Can you work these out from the model? Positions are in its coordinate system, mm. A direction names the side the tool comes from. Round coordinates to 2 decimals unless told otherwise and drop trailing zeros. Loops run counter-clockwise (first coordinate to the right, second up) from the corner with the lowest first, then second, coordinate; pieces in that order, holes last.
```python
from build123d import *

# Parameters (mm, degrees)
SKETCH1_R           = 2.5
BOSS_EXTRUDE1_DEPTH = 7.5


with BuildPart() as part:
    # Sketch1 → Boss-Extrude1 (new body)
    # profile 1 of 2: a face of its own
    with BuildSketch(Plane.XY):
        with BuildLine():
            ThreePointArc((47, 4), (55, 0), (47, -4))
            Line((47, -4), (-47, -4))
            ThreePointArc((-47, -4), (-55, 0), (-47, 4))
            Line((-47, 4), (47, 4))
        make_face()
        Circle(SKETCH1_R, mode=Mode.SUBTRACT)
        with BuildLine():
            ThreePointArc((52.5, 1.5), (52.207106781, 2.207106781), (51.5, 2.5))
            Line((51.5, 2.5), (48.5, 2.5))
            ThreePointArc((48.5, 2.5), (47.792893219, 2.207106781), (47.5, 1.5))
            Line((47.5, 1.5), (47.5, -1.5))
            ThreePointArc((47.5, -1.5), (47.792893219, -2.207106781), (48.5, -2.5))
            Line((48.5, -2.5), (51.5, -2.5))
            ThreePointArc((51.5, -2.5), (52.207106781, -2.207106781), (52.5, -1.5))
            Line((52.5, -1.5), (52.5, 1.5))
        make_face(mode=Mode.SUBTRACT)
        with BuildLine():
            Line((-52.5, -1.5), (-52.5, 1.5))
            ThreePointArc((-52.5, 1.5), (-52.207106781, 2.207106781), (-51.5, 2.5))
            Line((-51.5, 2.5), (-48.5, 2.5))
            ThreePointArc((-48.5, 2.5), (-47.792893219, 2.207106781), (-47.5, 1.5))
            Line((-47.5, 1.5), (-47.5, -1.5))
            ThreePointArc((-47.5, -1.5), (-47.792893219, -2.207106781), (-48.5, -2.5))
            Line((-48.5, -2.5), (-51.5, -2.5))
            ThreePointArc((-51.5, -2.5), (-52.207106781, -2.207106781), (-52.5, -1.5))
        make_face(mode=Mode.SUBTRACT)
    # profile 2 of 2: a face of its own
    with BuildSketch(Plane.XY):
        Circle(SKETCH1_R)
    extrude(amount=BOSS_EXTRUDE1_DEPTH)


solid = part.part
```
(1) Which directions (+Z, -Z, +X, -X, +Y, -Y) give clear straight access to the entire face, cutting with the end or side of a thin tool? Please do faces 1 (the flat face through (-1, 4, 4)), 2 (the flat face through (-50, -2.5, 4)), 3 (the flat face through (1, -4, 4)).
(2) Suppose I cut it at A-A (x = 50). Write out the boundary of the cut face in (y, z).
(3) If I drill on line 1 (Y direction, x = 3.5, z = 1); line 2 (X direction, y = -0.5, z = 5.25); line 3 (Y direction, x = 49, z = 4), over which ranges is the centre line in solid material (lowest first)?
(4) Suppose I cut it at D-D (x = -6). Write out the boundary of the cut face in (y, z).
(5) We'd pull the mould along X, two halves only. Please class faces 4 (the flat face through (1, 0, 7.5)), 5 (the flat face through (47.5, 0, 4)), 6 (the flat face through (52.5, 0, 4)): released by +X, released by -X, zero draft, split by the parting line, or undercut.
(6) Suppose I cut it at C-C (z = 5.5). Write out the boundary of the cut face in (x, y).
(7) Suppose I cut it at B-B (y = 0). Write out the boundary of the cut face in (x, z), then the cut area to 3 significant figures.
(8) For pin 1 (1 mm diameter, centred on x = 24.5, y = 3, fed in from -Z); pin 2 (2 mm diameter, centred on x = -20, z = 4, fed in from +Y), each with a flat end and sliding along its axis, tell me the tip position at first contact or that it passes through.
Check result:
1. face 1: +Z, -Z, +Y
1. face 2: +Z, -Z
1. face 3: +Z, -Z, -Y
2. outline: (-5, 0) - (-2.5, 0) - (-2.5, 7.5) - (-5, 7.5) - close; (2.5, 0) - (5, 0) - (5, 7.5) - (2.5, 7.5) - close
3. line 1: y = -4 to 4
3. line 2: x = -54.97 to -52.5, -47.5 to 47.5, 52.5 to 54.97
3. line 3: y = -4.9 to -2.5, 2.5 to 4.9
4. outline: (-4, 0) - (4, 0) - (4, 7.5) - (-4, 7.5) - close
5. face 4: zero draft
5. face 5: undercut
5. face 6: undercut
6. outline: (-47, -4) - (47, -4) arc R5 ccw (long way) to (47, 4) - (-47, 4) arc R5 ccw (long way) to start; hole (-52.5, -1.5) arc R1 ccw to (-51.5, -2.5) - (-48.5, -2.5) arc R1 ccw to (-47.5, -1.5) - (-47.5, 1.5) arc R1 ccw to (-48.5, 2.5) - (-51.5, 2.5) arc R1 ccw to (-52.5, 1.5) - close; hole (47.5, -1.5) arc R1 ccw to (48.5, -2.5) - (51.5, -2.5) arc R1 ccw to (52.5, -1.5) - (52.5, 1.5) arc R1 ccw to (51.5, 2.5) - (48.5, 2.5) arc R1 ccw to (47.5, 1.5) - close
7. outline: (-55, 0) - (-52.5, 0) - (-52.5, 7.5) - (-55, 7.5) - close; (-47.5, 0) - (47.5, 0) - (47.5, 7.5) - (-47.5, 7.5) - close; (52.5, 0) - (55, 0) - (55, 7.5) - (52.5, 7.5) - close
7. area: 750 mm2
8. pin 1: stops at z = 0
8. pin 2: stops at y = 4
